```python
from build123d import *

# Parameters (mm, degrees)
CROQUIS2_R              = 73.5
SALIENTE_EXTRUIR1_DEPTH = 14
CROQUIS6_R              = 70
SALIENTE_EXTRUIR4_DEPTH = 14
CROQUIS8_R              = 73.5
SALIENTE_EXTRUIR5_DEPTH = 14
CROQUIS10_R             = 21
CORTAR_EXTRUIR2_DEPTH   = 84
CROQUIS11_R             = 10.5
CORTAR_EXTRUIR3_DEPTH   = 84


with BuildPart() as part:
    # Croquis2 → Saliente-Extruir1 (new body)
    with BuildSketch(Plane.XY):
        Circle(CROQUIS2_R)
    extrude(amount=SALIENTE_EXTRUIR1_DEPTH)

    # Croquis6 → Saliente-Extruir4 (add)
    with BuildSketch(Plane.XY):
        Circle(CROQUIS6_R)
    extrude(amount=-SALIENTE_EXTRUIR4_DEPTH)

    # Croquis8 → Saliente-Extruir5 (add)
    with BuildSketch(Plane(origin=(0, 0, -14), x_dir=(-1, 0, 0), z_dir=(0, 0, -1))):
        Circle(CROQUIS8_R)
    extrude(amount=SALIENTE_EXTRUIR5_DEPTH)

    # Croquis10 → Cortar-Extruir2 (cut)
    with BuildSketch(Plane.XY.offset(14)):
        Circle(CROQUIS10_R)
    extrude(amount=-CORTAR_EXTRUIR2_DEPTH, mode=Mode.SUBTRACT)

    # Croquis11 → Cortar-Extruir3 (cut)
    with BuildSketch(Plane(origin=(0, 0, -28), x_dir=(-1, 0, 0), z_dir=(0, 0, -1))):
        with Locations((52.5, 0)):
            Circle(CROQUIS11_R)
    extrude(amount=-CORTAR_EXTRUIR3_DEPTH, mode=Mode.SUBTRACT)


solid = part.part
```
Geometry check sheet. Reference: the model listing, model coordinates, mm. A direction names the side the tool comes from. Coordinates: 2 decimals unless noted, no trailing zeros. Order: outer loops, then holes, each group sorted by start corner. A loop starts at its lowest first (then second) coordinate and runs counter-clockwise, first axis right, second up.
Q1. Draft check along Z on faces 1 (the face through (15, -15, 14)), 2 (the face through (-65, -27, -14)), 3 (the face through (-15.933, -71.752, 6.902)). Enter one of: released by +Z, released by -Z, zero draft, split by the parting line, or undercut.
Reply:
face 1: released by +Z
face 2: undercut
face 3: zero draft
Q2. Thickness scan on probe 1 along Y at (x, z) = (0, -12.5); probe 2 along Z at (x, y) = (64, -30); probe 3 along X at (y, z) = (14, -17.5). Record the ranges inside material, lowest first.
Reply:
probe 1: y = -70 to -21, 21 to 70
probe 2: z = -28 to -14, 0 to 14
probe 3: x = -72.15 to -15.65, 15.65 to 72.15
Q3. Sectioned sample at A-A on y = 0. Record the cut outline in (x, z), and give its area (3 significant figures).
Reply:
outline: (-73.5, -28) - (-63, -28) - (-63, 14) - (-73.5, 14) - (-73.5, 0) - (-70, 0) - (-70, -14) - (-73.5, -14) - close; (-42, -28) - (-21, -28) - (-21, 14) - (-42, 14) - close; (21, -28) - (73.5, -28) - (73.5, -14) - (70, -14) - (70, 0) - (73.5, 0) - (73.5, 14) - (21, 14) - close
area: 3,430 mm2
Q4. Sectioned sample at D-D on z = 7. Record the cut outline in (x, y), and give its area (3 significant figures).
Reply:
outline: circle Ø147 at (0, 0); hole circle Ø21 at (-52.5, 0); hole circle Ø42 at (0, 0)
area: 15,200 mm2
Q5. Sectioned sample at C-C on y = -19. Record the cut outline in (x, z), and give its area (3 significant figures).
Reply:
outline: (-71, -28) - (-8.94, -28) - (-8.94, 14) - (-71, 14) - (-71, 0) - (-67.37, 0) - (-67.37, -14) - (-71, -14) - close; (8.94, -28) - (71, -28) - (71, -14) - (67.37, -14) - (67.37, 0) - (71, 0) - (71, 14) - (8.94, 14) - close
area: 5,110 mm2
Q6. Tool access check on faces 4 (the face through (-42, 0, -7)), 5 (the face through (-55.55, -42.594, -6.902)). Record the directions out of +Z, -Z, +X, -X, +Y, -Y that give a thin tool (end or side, any length) a straight path to the whole face; none if there is none.
Reply:
face 4: +Z, -Z
face 5: none
Q7. Depth check by flat-ended pin: pin 1 Ø5 at (y, z) = (57.5, -20.5) entering from +X; pin 2 Ø4 at (x, z) = (-31, -5) entering from -Y; pin 3 Ø4 at (y, z) = (-17, 4.5) entering from +X. Enter the tip coordinate at first touch or a pass-through.
Reply:
pin 1: stops at x = 48.76
pin 2: stops at y = -63.71
pin 3: stops at x = 71.95
Q8. Sectioned sample at B-B on x = 0. Record the cut outline in (y, z).
Reply:
outline: (-73.5, -28) - (-21, -28) - (-21, 14) - (-73.5, 14) - (-73.5, 0) - (-70, 0) - (-70, -14) - (-73.5, -14) - close; (21, -28) - (73.5, -28) - (73.5, -14) - (70, -14) - (70, 0) - (73.5, 0) - (73.5, 14) - (21, 14) - close
